Geometry: see drawing. Coordinates: mm, zero at the bounding-box minimum. Round coordinates to 2 decimals unless told otherwise and drop trailing zeros. Write each loop counter-clockwise with the first axis right and the second up, starting at its lowest first coordinate (ties: lowest second). Pieces come first, ordered by that corner, then holes. Notation, with made-up numbers: M 0.25,27 L 20.25,27 A28 cw 20.25,61 Z; hole C 80.5,36 d8. An arc over 180 degrees is marked long. Use one line per item in the form item = value. Start each with the question number.
Item 1: Pin query (flat end, axial travel): pin 1 Ø3 at (y, z) = (0.5, 4) entering from -X. Return the tip coordinate at first contact, or that it passes through.
Item 2: Section query C-C (z = 3.75). Return loops of the section in (x, y).
Item 3: Section query D-D (y = 4.45). Return loops of the section in (x, z), and give its area (3 significant figures).
Item 4: Ray query, probe 1 along Z at (x, y) = (0.3, 2.5); probe 2 along Z at (x, y) = (0.15, 4.8); probe 3 along Y at (x, z) = (0.6, 4.75). Return the intervals inside material, ascending.
Item 5: Pull-direction query (Y, two-part tool) for the marked faces 1, 2 and 3; classes: pulls with the +Y half, pulls with the -Y half, needs draft (parallel to the pull), parting line crosses it, or undercut.
Item 6: Section query A-A (y = 3.1). Return loops of the section in (x, z), and give its area (3 significant figures).
Item 7: Section query B-B (x = 0.35). Return loops of the section in (y, z), and give its area (3 significant figures).
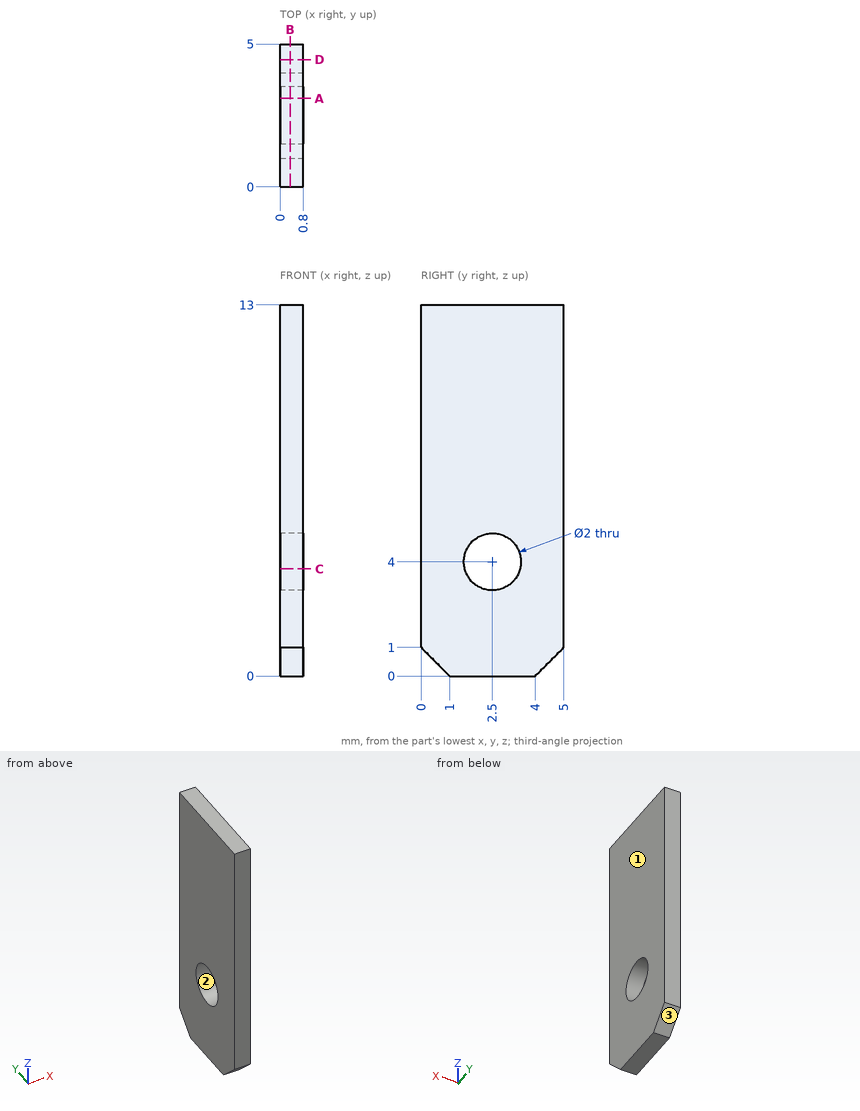
Working result:
q1.pin_1 = 0
q2.outline = M 0,0 L 0.8,0 L 0.8,1.53 L 0,1.53 Z; M 0,3.47 L 0.8,3.47 L 0.8,5 L 0,5 Z
q3.outline = M 0,0.45 L 0.8,0.45 L 0.8,13 L 0,13 Z
q3.area = 10.0 mm²
q4.probe_1 = 0 to 3, 5 to 13
q4.probe_2 = 0.8 to 13
q4.probe_3 = 0 to 1.84, 3.16 to 5
q5.face_1 = needs draft
q5.face_2 = undercut
q5.face_3 = pulls with the +Y half
q6.outline = M 0,0 L 0.8,0 L 0.8,3.2 L 0,3.2 Z; M 0,4.8 L 0.8,4.8 L 0.8,13 L 0,13 Z
q6.area = 9.12 mm²
q7.outline = M 0,1 L 1,0 L 4,0 L 5,1 L 5,13 L 0,13 Z; hole C 2.5,4 d2
q7.area = 60.9 mm²
